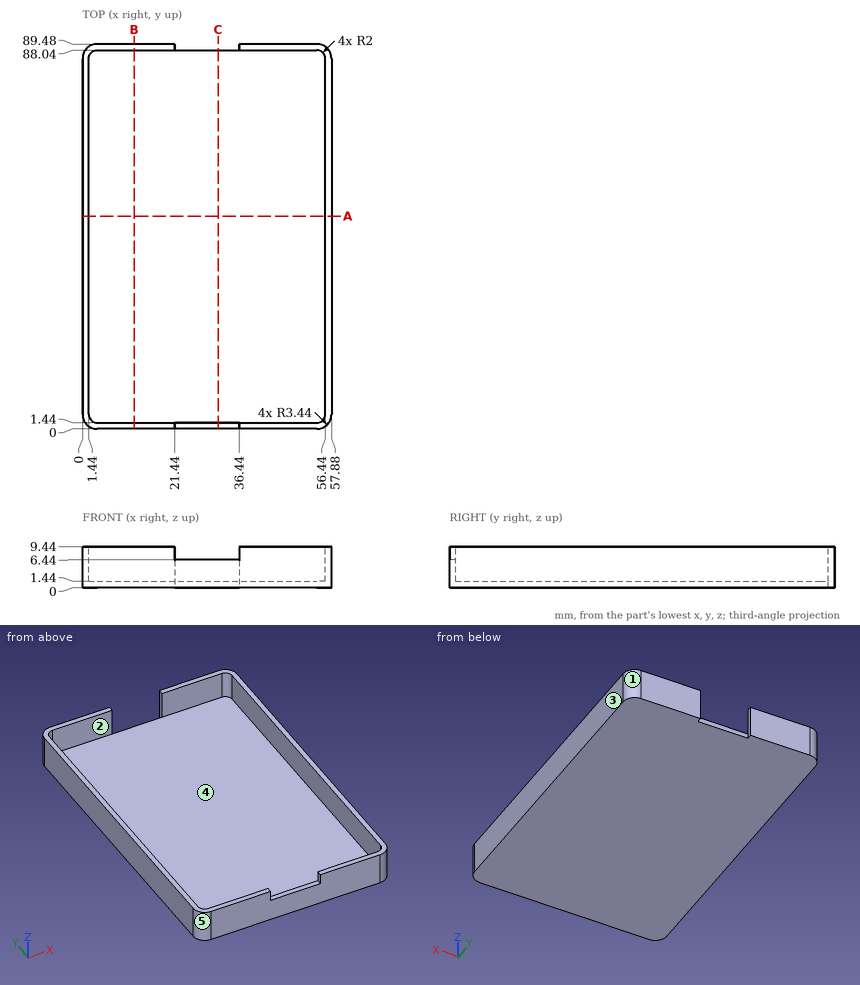
Drawing for the job (mm, zero at the part's lowest x, y, z). A direction names the side the tool comes from. Round coordinates to 2 decimals unless told otherwise and drop trailing zeros. Order: outer loops, then holes, each group sorted by start corner. A loop starts at its lowest first (then second) coordinate and runs counter-clockwise, first axis right, second up.
Item 1: Pin check, flat tips, straight feed: pin 1 (1.5 mm diameter, centred on x = 32, y = 16.5, fed in from +Z); pin 2 (1.6 mm diameter, centred on x = 31, z = 0.5, fed in from +Y); pin 3 (1.2 mm diameter, centred on x = 25.5, y = 1, fed in from +Z). Stop position of each tip, or through.
Item 2: Saw through at A-A on y = 49.5. Write the cut outline in (x, z).
Item 3: Saw through at B-B on x = 12. Write the cut outline in (y, z).
Item 4: Mould opens along Y. For the marked faces 3, 4 and 5 say: pulls with the +Y half, pulls with the -Y half, needs draft (parallel to the pull), parting line crosses it, or undercut.
Item 5: Tool access for the marked faces 1 and 2: list every direction of +Z, -Z, +X, -X, +Y, -Y with a clear straight run to the whole face (end or side of a thin tool).
Item 6: Saw through at C-C on x = 31.5. Write the cut outline in (y, z), then the cut area to 3 significant figures.
Item 7: Probe line 1 along X through (y, z) = (29.5, 1.75); line 2 along Y through (x, z) = (17, 8.25); line 3 along Z through (x, y) = (40, 82.5). List the from-to ranges inside material, lowest first.
Reported:
1. pin 1: stops at z = 1.44
1. pin 2: stops at y = 88.04
1. pin 3: stops at z = 6.44
2. outline: (0, 0) - (57.88, 0) - (57.88, 9.44) - (56.44, 9.44) - (56.44, 1.44) - (1.44, 1.44) - (1.44, 9.44) - (0, 9.44) - close
3. outline: (0, 0) - (89.48, 0) - (89.48, 9.44) - (88.04, 9.44) - (88.04, 1.44) - (1.44, 1.44) - (1.44, 9.44) - (0, 9.44) - close
4. face 3: needs draft
4. face 4: undercut
4. face 5: pulls with the -Y half
5. face 1: +Z, -Z, +X, +Y
5. face 2: +Z
6. outline: (0, 0) - (88.04, 0) - (88.04, 1.44) - (1.44, 1.44) - (1.44, 6.44) - (0, 6.44) - close
6. area: 134 mm2
7. line 1: x = 0 to 1.44, 56.44 to 57.88
7. line 2: y = 0 to 1.44, 88.04 to 89.48
7. line 3: z = 0 to 1.44
